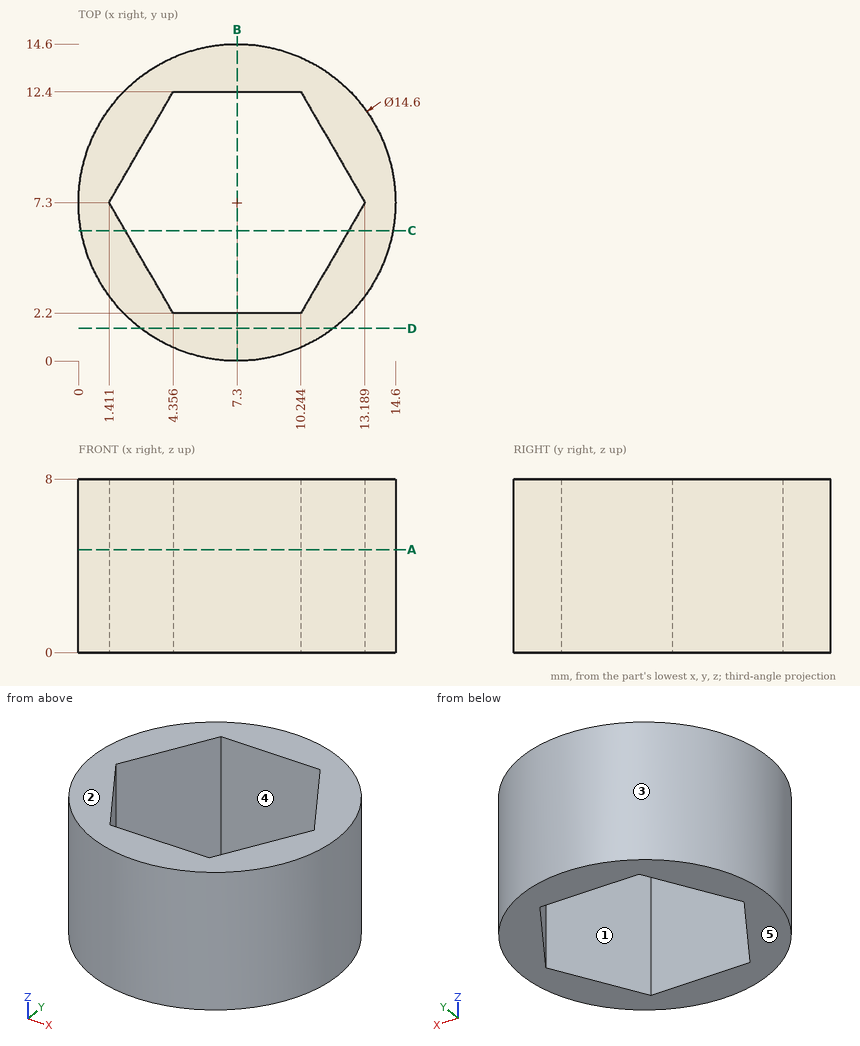
Design review of the part shown in the three views and the two pictorial views. Dimensions are in mm from the part's minimum x, y and z. A direction names the side the tool comes from. Give positions to 0.01 mm unless a question says otherwise; leave off trailing zeros. Loops run counter-clockwise (first coordinate to the right, second up) from the corner with the lowest first, then second, coordinate; pieces in that order, holes last. Notation, with made-up numbers: M 0,61.25 L 19,61.25 A18 cw 19,86.25 Z; hole C 10.25,37 d2. An arc over 180 degrees is marked long. Answer as a JSON object with one key per item and string values. Group by question number.
Q1. Insertion check: P1, Ø1, axis at y = 11.5, z = 2, coming from the -X side; P2, Ø2, axis at x = 7, y = 10, coming from the +Z side; P3, Ø1.5, axis at x = 5.5, z = 2, coming from the -Y side; P4, Ø1.5, axis at x = 12.5, z = 4, coming from the +Y side. Each pin has a flat end and moves straight along its axis. Give the tip position at first contact, or say it passes through.
Q2. Add section D-D on y = 1.5. Give the boundary of the cut face in (x, z).
Q3. Add section A-A on z = 4.75. Give the boundary of the cut face in (x, y) (1 decimal).
Q4. Add section B-B on x = 7.3. Give the boundary of the cut face in (y, z), and give its area (3 significant figures).
Q5. For probe 1 along Y at (x, z) = (7.5, 6); probe 2 along Y at (x, z) = (12.25, 1.25) (1 decimal); probe 3 along X at (y, z) = (7.75, 2.25) (1 decimal), list the stretches that pass through material, from the lowest coordinate up. Write a range as [from, to].
Q6. Add section C-C on y = 6. Give the boundary of the cut face in (x, z).
Q7. Tool access review of the marked faces 1 and 2: name each direction out of +Z, -Z, +X, -X, +Y, -Y from which nothing blocks a thin tool from reaching the whole face with its end or side.
Q8. Mouldability with a two-part tool opening along Y and no side actions: class the marked faces 3, 4 and 5 as +Y half, -Y half, draft (parallel to the pull), parting line (faces both ways), or undercut.
Checked values:
{
 "1": {"P1": "x = 1.01", "P2": "through", "P3": "y = 0.08", "P4": "y = 13.09"},
 "2": {"outline": "M 2.87,0 L 11.73,0 L 11.73,8 L 2.87,8 Z"},
 "3": {"outline": "C 7.3,7.3 d14.6; hole M 1.4,7.3 L 4.4,2.2 L 10.2,2.2 L 13.2,7.3 L 10.2,12.4 L 4.4,12.4 Z"},
 "4": {"outline": "M 0,0 L 2.2,0 L 2.2,8 L 0,8 Z; M 12.4,0 L 14.6,0 L 14.6,8 L 12.4,8 Z", "area": "35.2 mm²"},
 "5": {"probe 1": "[0, 2.2], [12.4, 14.6]", "probe 2": "[1.9, 5.7], [8.9, 12.7]", "probe 3": "[0, 1.7], [12.9, 14.6]"},
 "6": {"outline": "M 0.12,0 L 2.16,0 L 2.16,8 L 0.12,8 Z; M 12.44,0 L 14.48,0 L 14.48,8 L 12.44,8 Z"},
 "7": {"face 1": "+Z, -Z", "face 2": "+Z, +X, -X, +Y, -Y"},
 "8": {"face 3": "parting line", "face 4": "undercut", "face 5": "draft"}
}
